The model under review builds one solid part; all positions refer to its coordinate system, in mm. Face numbers are marked on the shaded views. A direction names the side the tool comes from. Round coordinates to 2 decimals unless told otherwise and drop trailing zeros. Loops run counter-clockwise (first coordinate to the right, second up) from the corner with the lowest first, then second, coordinate; pieces in that order, holes last. Notation, with made-up numbers: M 18,51.5 L 60,51.5 A25 ccw 60,77.5 Z; hole C 41,74 d8. An arc over 180 degrees is marked long. Return JSON: item names as keys, results as strings. Group by question number.
Q1. To check wall thickness, follow line 1 along X through (y, z) = (17.5, -6); line 2 along Z through (x, y) = (9.75, 3); line 3 along Y through (x, z) = (-0.75, -14.5). State the ranges of each line that lie inside material, in increasing order.
Q2. Clearance check with flat-ended pins moving along their axes: pin 1 Ø6 at (y, z) = (15.5, -10) entering from -X; pin 2 Ø1.2 at (x, z) = (-0.5, -15) entering from +Y; pin 3 Ø4.5 at (y, z) = (33.5, -11.5) entering from +X. State where each tip first meets the part, or that it passes through.
Q3. Consider section B-B (x = 8.75). State the section outline as (y, z) points.
Q4. Consider section C-C (z = -14.5). State the section outline as (x, y) points, and give its area (3 significant figures).
Q5. For the marked faces 1, 2, 3, 4 and 5, list the 3-axis set-ups (+Z, -Z, +X, -X, +Y, -Y) from which the entire face can be reached by the end or side of a thin tool; tool diameter is ignored.
Q6. Consider section A-A (y = 14.5). State the section outline as (x, z) points, and give its area (3 significant figures).
from build123d import *

# Parameters (mm, degrees)
SKETCH1_W           = 15
SKETCH1_H           = 80
BOSS_EXTRUDE1_DEPTH = 5
SKETCH3_W           = 23
SKETCH3_H           = 60
BOSS_EXTRUDE3_DEPTH = 4
SKETCH5_W           = 4
SKETCH5_H           = 50
BOSS_EXTRUDE5_DEPTH = 15
SKETCH6_W           = 15
SKETCH6_H           = 5
CUT_EXTRUDE1_DEPTH  = 80
SKETCH7_W           = 4
SKETCH7_H           = 15
CUT_EXTRUDE2_DEPTH  = 15


with BuildPart() as part:
    # Sketch1 → Boss-Extrude1 (new body)
    with BuildSketch(Plane(origin=(0, 0, 0), x_dir=(1, 0, 0), z_dir=(0, 1, 0))):
        with Locations((7.5, -40)):
            Rectangle(SKETCH1_W, SKETCH1_H)
    extrude(amount=BOSS_EXTRUDE1_DEPTH)

    # Sketch3 → Boss-Extrude3 (add)
    with BuildSketch(Plane(origin=(0, 0, 0), x_dir=(-1, 0, 0), z_dir=(0, 0, -1))):
        with Locations((-7.5, 30)):
            Rectangle(SKETCH3_W, SKETCH3_H)
    extrude(amount=BOSS_EXTRUDE3_DEPTH)

    # Sketch5 → Boss-Extrude5 (add)
    with BuildSketch(Plane(origin=(0, 0, -4), x_dir=(-1, 0, 0), z_dir=(0, 0, -1))):
        with Locations((-0.25, 35)):
            Rectangle(SKETCH5_W, SKETCH5_H)
    extrude(amount=BOSS_EXTRUDE5_DEPTH)

    # Sketch6 → Cut-Extrude1 (cut)
    with BuildSketch(Plane.XY.offset(80)):
        with Locations((7.5, 2.5)):
            Rectangle(SKETCH6_W, SKETCH6_H)
    extrude(amount=-CUT_EXTRUDE1_DEPTH, mode=Mode.SUBTRACT)

    # Sketch7 → Cut-Extrude2 (cut)
    with BuildSketch(Plane(origin=(0, 0, -19), x_dir=(-1, 0, 0), z_dir=(0, 0, -1))):
        with Locations((-0.25, 52.5)):
            Rectangle(SKETCH7_W, SKETCH7_H)
    extrude(amount=-CUT_EXTRUDE2_DEPTH, mode=Mode.SUBTRACT)


solid = part.part
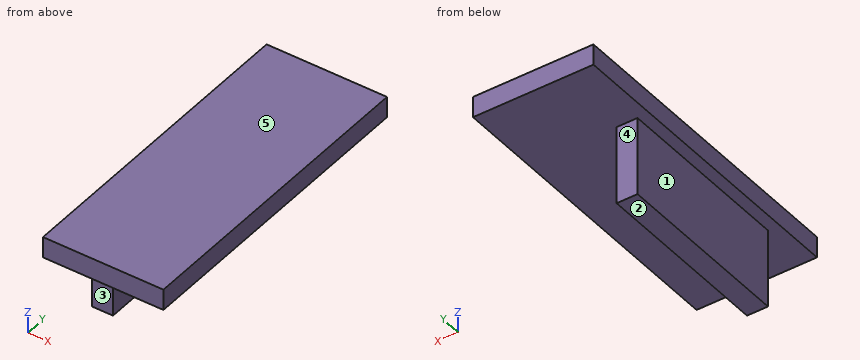
Values:
{
 "1": {"line 1": "x = -1.75 to 2.25", "line 2": "z = -4 to 0", "line 3": "y = 10 to 45"},
 "2": {"pin 1": "stops at x = -1.75", "pin 2": "stops at y = 45", "pin 3": "stops at x = 2.25"},
 "3": {"outline": "M 0,-4 L 60,-4 L 60,0 L 0,0 Z"},
 "4": {"outline": "M -1.75,10 L 2.25,10 L 2.25,45 L -1.75,45 Z", "area": "140 mm2"},
 "5": {"face 1": "-Z, -X, +Y, -Y", "face 2": "-Z, +X, -X, +Y, -Y", "face 3": "-Z, +X, -X, -Y", "face 4": "-Z, +X, -X, +Y", "face 5": "+Z, +X, -X, +Y, -Y"},
 "6": {"outline": "M -4,-4 L -1.75,-4 L -1.75,-19 L 2.25,-19 L 2.25,-4 L 19,-4 L 19,0 L -4,0 Z", "area": "152 mm2"}
}
